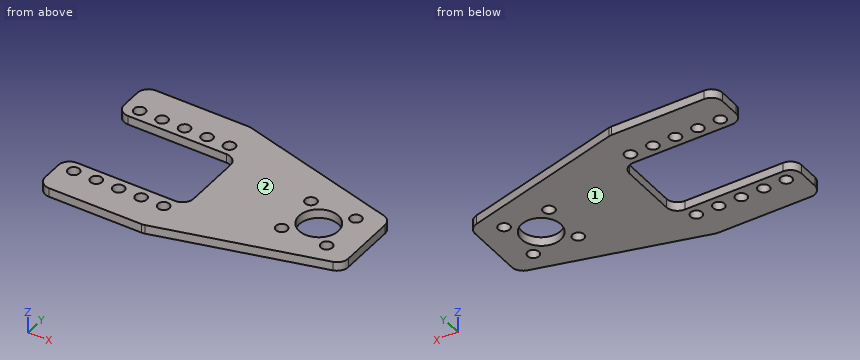
from build123d import *

# Parameters (mm, degrees)
SKETCH1_R           = 7
SKETCH1_R_2         = 2.05
BOSS_EXTRUDE2_DEPTH = 3.175
FILLET2_R           = 4


with BuildPart() as part:
    # Sketch1 → Boss-Extrude2 (new body)
    with BuildSketch(Plane.XY):
        Polygon((37.5, -43.175), (0, -43.175), (0, -28), (43, -28), (43, 0), (0, 0), (0, 15.175), (37.5, 15.175), (98, -0.934242296), (98, -27.065757704), align=None)
        with Locations((81, -14)):
            Circle(SKETCH1_R, mode=Mode.SUBTRACT)
        with Locations((13.5, -32)):
            Circle(SKETCH1_R_2, mode=Mode.SUBTRACT)
        with Locations((29.5, -32)):
            Circle(SKETCH1_R_2, mode=Mode.SUBTRACT)
        with Locations((73, -6)):
            Circle(SKETCH1_R_2, mode=Mode.SUBTRACT)
        with Locations((89, -6)):
            Circle(SKETCH1_R_2, mode=Mode.SUBTRACT)
        with Locations((89, -22)):
            Circle(SKETCH1_R_2, mode=Mode.SUBTRACT)
        with Locations((73, -22)):
            Circle(SKETCH1_R_2, mode=Mode.SUBTRACT)
        with Locations((5.5, 4)):
            Circle(SKETCH1_R_2, mode=Mode.SUBTRACT)
        with Locations((13.5, 4)):
            Circle(SKETCH1_R_2, mode=Mode.SUBTRACT)
        with Locations((21.5, 4)):
            Circle(SKETCH1_R_2, mode=Mode.SUBTRACT)
        with Locations((29.5, 4)):
            Circle(SKETCH1_R_2, mode=Mode.SUBTRACT)
        with Locations((37.5, 4)):
            Circle(SKETCH1_R_2, mode=Mode.SUBTRACT)
        with Locations((37.5, -32)):
            Circle(SKETCH1_R_2, mode=Mode.SUBTRACT)
        with Locations((21.5, -32)):
            Circle(SKETCH1_R_2, mode=Mode.SUBTRACT)
        with Locations((5.5, -32)):
            Circle(SKETCH1_R_2, mode=Mode.SUBTRACT)
    extrude(amount=BOSS_EXTRUDE2_DEPTH)

    # Fillet2
    fillet2_edges = [part.edges().sort_by_distance(p)[0] for p in [
        (0, -43.175, 1.5875),
        (0, -28, 1.5875),
        (43, -28, 1.5875),
        (43, 0, 1.5875),
        (0, 0, 1.5875),
        (0, 15.175, 1.5875),
        (37.5, 15.175, 1.5875),
        (98, -0.934242296, 1.5875),
        (98, -27.065757704, 1.5875),
        (37.5, -43.175, 1.5875),
    ]]
    fillet(fillet2_edges, radius=FILLET2_R)


solid = part.part
CAD build for the part. Positions are in the model's coordinates, mm. Face numbers are marked on the shaded views. Round coordinates to 2 decimals unless told otherwise and drop trailing zeros. Order: outer loops, then holes, each group sorted by start corner. A loop starts at its lowest first (then second) coordinate and runs counter-clockwise, first axis right, second up. Notation, with made-up numbers: (-5.5, -26) -> (19.5, -26) arc R19 ccw to (19.5, -14) -> close; hole circle Ø1 at (22, 84.5). An arc over 180 degrees is marked (long way). Write each question's results on one line, items separated by ' | '.
1. Wall check: line 1 along Y through (x, z) = (29.5, 1.5) (3 decimals); line 2 along X through (y, z) = (-13.5, 0.3); line 3 along Y through (x, z) = (23, 2.85) (3 decimals). Give the ranges that are in metal, low to high. Write a range as [from, to].
Findings below:
line 1: y = [-43.175, -34.05], [-29.95, -28], [0, 1.95], [6.05, 15.175] | line 2: x = [43, 74.02], [87.98, 98] | line 3: y = [-43.175, -33.397], [-30.603, -28], [0, 2.603], [5.397, 15.175]
2. Cut at C-C (y = -6). Give the cut face in (x, z) (3 decimals).
Findings below:
outline: (43, 0) -> (70.95, 0) -> (70.95, 3.175) -> (43, 3.175) -> close; (75.05, 0) -> (86.95, 0) -> (86.95, 3.175) -> (75.05, 3.175) -> close; (91.05, 0) -> (98, 0) -> (98, 3.175) -> (91.05, 3.175) -> close
3. Cut at A-A (y = -14). Give the cut face in (x, z) (3 decimals), plus the area to 3 significant figures.
Findings below:
outline: (43, 0) -> (74, 0) -> (74, 3.175) -> (43, 3.175) -> close; (88, 0) -> (98, 0) -> (98, 3.175) -> (88, 3.175) -> close | area: 130 mm²
4. Flat gauge pin, fed straight in: P1, Ø1, axis at y = -11.5, z = 2, coming from the -X side. Where does the tip first touch, or does it go through?
Findings below:
P1: stops at x = 43
5. Cut at B-B (x = 5.5). Give the cut face in (y, z) (3 decimals), plus the area to 3 significant figures.
Findings below:
outline: (-43.175, 0) -> (-34.05, 0) -> (-34.05, 3.175) -> (-43.175, 3.175) -> close; (-29.95, 0) -> (-28, 0) -> (-28, 3.175) -> (-29.95, 3.175) -> close; (0, 0) -> (1.95, 0) -> (1.95, 3.175) -> (0, 3.175) -> close; (6.05, 0) -> (15.175, 0) -> (15.175, 3.175) -> (6.05, 3.175) -> close | area: 70.3 mm²
6. Cut at D-D (x = 89). Give the cut face in (y, z) (3 decimals).
Findings below:
outline: (-29.462, 0) -> (-24.05, 0) -> (-24.05, 3.175) -> (-29.462, 3.175) -> close; (-19.95, 0) -> (-8.05, 0) -> (-8.05, 3.175) -> (-19.95, 3.175) -> close; (-3.95, 0) -> (1.462, 0) -> (1.462, 3.175) -> (-3.95, 3.175) -> close
7. Pull direction Z, two halves, no side cores. Call the marked faces 1 and 2: pulls with the +Z half, pulls with the -Z half, needs draft (parallel to the pull), parting line crosses it, or undercut.
Findings below:
face 1: pulls with the -Z half | face 2: pulls with the +Z half
